Design review of the part built by this model. Coordinates are the model's own, in mm. A direction names the side the tool comes from. Give positions to 0.01 mm unless a question says otherwise; leave off trailing zeros. Write each loop counter-clockwise with the first axis right and the second up, starting at its lowest first coordinate (ties: lowest second). Pieces come first, ordered by that corner, then holes.
```python
from build123d import *

# Parameters (mm, degrees)
SKETCH1_W           = 100
SKETCH1_H           = 40
BOSS_EXTRUDE1_DEPTH = 10
SKETCH2_W           = 100
SKETCH2_H           = 10
BOSS_EXTRUDE2_DEPTH = 90
SKETCH3_R           = 3.95
BOSS_EXTRUDE3_DEPTH = 50
SKETCH4_R           = 2
CUT_EXTRUDE1_DEPTH  = 50


with BuildPart() as part:
    # Sketch1 → Boss-Extrude1 (new body)
    with BuildSketch(Plane.XY):
        Rectangle(SKETCH1_W, SKETCH1_H)
    extrude(amount=BOSS_EXTRUDE1_DEPTH)

    # Sketch2 → Boss-Extrude2 (add)
    with BuildSketch(Plane.XY.offset(10)):
        with Locations((0, -15)):
            Rectangle(SKETCH2_W, SKETCH2_H)
    extrude(amount=BOSS_EXTRUDE2_DEPTH)

    # Sketch3 → Boss-Extrude3 (add)
    with BuildSketch(Plane.XZ.offset(20)):
        with Locations(Location((0, 60, 0), (0, 0, 90))):
            Circle(SKETCH3_R)
    extrude(amount=BOSS_EXTRUDE3_DEPTH)

    # Sketch4 → Cut-Extrude1 (cut)
    with BuildSketch(Plane.XY.offset(10)):
        with Locations((-25, 5)):
            Circle(SKETCH4_R)
        with Locations((25, 5)):
            Circle(SKETCH4_R)
    extrude(amount=-CUT_EXTRUDE1_DEPTH, mode=Mode.SUBTRACT)


solid = part.part
```
(1) Consider section B-B, the plane y = 5. Give the boundary of the cut face in (x, z).
Resolved:
outline: (-50, 0) - (-27, 0) - (-27, 10) - (-50, 10) - close; (-23, 0) - (23, 0) - (23, 10) - (-23, 10) - close; (27, 0) - (50, 0) - (50, 10) - (27, 10) - close
(2) Mouldability with a two-part tool opening along Y and no side actions: class faces 4 (the face through (-1, 0, 0)), 5 (the face through (-27, 5, 5)), 6 (the face through (23, 5, 5)), 7 (the face through (0, -70, 60)) as pulls with the +Y half, pulls with the -Y half, needs draft (parallel to the pull), parting line crosses it, or undercut.
Resolved:
face 4: needs draft
face 5: undercut
face 6: undercut
face 7: pulls with the -Y half
(3) Tool access review of faces 1 (the face through (-0.174, -44.65, 56.054)), 2 (the face through (-1, -10, 54)), 3 (the face through (-1, -15, 100)): name each direction out of +Z, -Z, +X, -X, +Y, -Y from which nothing blocks a thin tool from reaching the whole face with its end or side.
Resolved:
face 1: -Y
face 2: +Z, +X, -X, +Y
face 3: +Z, +X, -X, +Y, -Y
(4) To check wall thickness, follow L1, parallel to Y at x = 25, z = 5; L2, parallel to Y at x = 24, z = 11; L3, parallel to Z at x = -28.5, y = -8. State the ranges of each line that lie inside material, in increasing order.
Resolved:
L1: y = -20 to 3, 7 to 20
L2: y = -20 to -10
L3: z = 0 to 10
(5) Consider section A-A, the plane x = -25. Give the boundary of the cut face in (y, z).
Resolved:
outline: (-20, 0) - (3, 0) - (3, 10) - (-10, 10) - (-10, 100) - (-20, 100) - close; (7, 0) - (20, 0) - (20, 10) - (7, 10) - close
(6) Consider section C-C, the plane z = 60. Give the boundary of the cut face in (x, y).
Resolved:
outline: (-50, -20) - (-3.95, -20) - (-3.95, -70) - (3.95, -70) - (3.95, -20) - (50, -20) - (50, -10) - (-50, -10) - close
(7) Clearance check with flat-ended pins moving along their axes: P1, Ø8, axis at x = 37.5, z = 76, coming from the +Y side; P2, Ø3, axis at x = -29, z = 54, coming from the -Y side; P3, Ø24, axis at x = -0.5, y = 5, coming from the +Z side. State where each tip first meets the part, or that it passes through.
Resolved:
P1: stops at y = -10
P2: stops at y = -20
P3: stops at z = 10
(8) Consider section D-D, the plane x = 0. Give the boundary of the cut face in (y, z), then the cut area to 4 significant figures.
Resolved:
outline: (-70, 56.05) - (-20, 56.05) - (-20, 0) - (20, 0) - (20, 10) - (-10, 10) - (-10, 100) - (-20, 100) - (-20, 63.95) - (-70, 63.95) - close
area: 1,695 mm2
